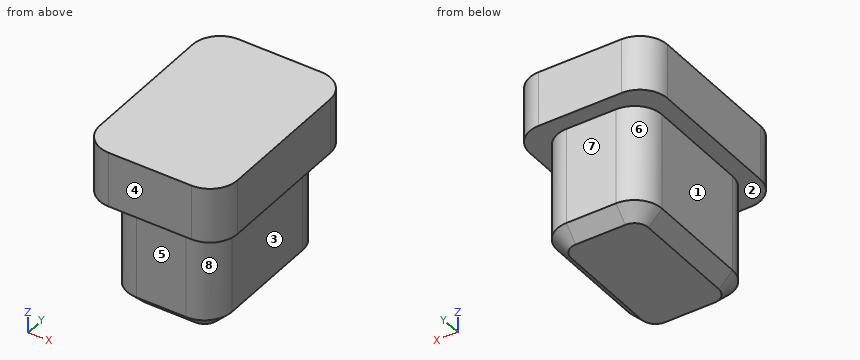
Autodesk Inventor part; units mm, degrees
ref_plane "YZ Plane" through (0, 0, 0) normal (1, 0, 0) x (0, 1, 0)
ref_plane "XZ Plane" through (0, 0, 0) normal (0, 1, 0) x (-1, 0, 0)
ref_plane "XY Plane" through (0, 0, 0) normal (0, 0, 1) x (1, 0, 0)
sketch "Sketch1" plane through (0, 0, 0) normal (0, 0, 1) x (1, 0, 0)
  line L0 (-0.9, 2.9) -> (0.9, 2.9)
  line L1 (1.9, 1.9) -> (1.9, -1.9)
  line L2 (0.9, -2.9) -> (-0.9, -2.9)
  line L3 (-1.9, -1.9) -> (-1.9, 1.9)
  arc A0 (1.9, 1.9) -> (0.9, 2.9) centre (0.9, 1.9) ccw
  arc A1 (0.9, -2.9) -> (1.9, -1.9) centre (0.9, -1.9) ccw
  arc A2 (-1.9, -1.9) -> (-0.9, -2.9) centre (-0.9, -1.9) ccw
  arc A3 (-0.9, 2.9) -> (-1.9, 1.9) centre (-0.9, 1.9) ccw
  point P0 (0, 0)
  point P1 (0, 2.9)
  point P2 (-1.9, 0)
  dimension "d1" = 3.8
  dimension "d2" = 5.8
  dimension "d3" = 1
extrude "Extrusion1" add sketch "Sketch1" along normal blind 4
sketch "Sketch2" plane through (0, 0, 4) normal (0, 0, 1) x (1, 0, 0)
  line L0 (-1.5, 3.5) -> (1.5, 3.5)
  line L1 (2.5, 2.5) -> (2.5, -2.5)
  line L2 (1.5, -3.5) -> (-1.5, -3.5)
  line L3 (-2.5, -2.5) -> (-2.5, 2.5)
  arc A0 (2.5, 2.5) -> (1.5, 3.5) centre (1.5, 2.5) ccw
  arc A1 (-2.5, -2.5) -> (-1.5, -3.5) centre (-1.5, -2.5) ccw
  arc A2 (1.5, -3.5) -> (2.5, -2.5) centre (1.5, -2.5) ccw
  arc A3 (-1.5, 3.5) -> (-2.5, 2.5) centre (-1.5, 2.5) ccw
  point P0 (0, 0)
  point P1 (-2.5, 3.5)
  point P2 (2.5, -3.5)
  point P3 (2.5, 3.5)
  point P4 (0, 3.5)
  point P5 (2.5, 0)
  dimension "d6" = 5
  dimension "d7" = 7
  dimension "d9" = 1
extrude "Extrusion2" add sketch "Sketch2" along normal blind 2
chamfer "Chamfer1" distance 0.5 angle 45 8 edges at (-1.9, 0, 0) (-1.6071, -2.6071, 0) (0, -2.9, 0) (1.6071, -2.6071, 0) (1.9, 0, 0) (1.6071, 2.6071, 0) (0, 2.9, 0) (-1.6071, 2.6071, 0)
properties part number "Button_Extender"
The model under review builds one solid part; all positions refer to its coordinate system, in mm. Face numbers are marked on the shaded views. A direction names the side the tool comes from. Round coordinates to 2 decimals unless told otherwise and drop trailing zeros. Order: outer loops, then holes, each group sorted by start corner. A loop starts at its lowest first (then second) coordinate and runs counter-clockwise, first axis right, second up.
(1) Take a section at A-A, the plane z = 4.4. State the section outline as (x, y) points, plus the area to 3 significant figures.
Working result:
outline: (-2.5, -2.5) arc R1 ccw to (-1.5, -3.5) - (1.5, -3.5) arc R1 ccw to (2.5, -2.5) - (2.5, 2.5) arc R1 ccw to (1.5, 3.5) - (-1.5, 3.5) arc R1 ccw to (-2.5, 2.5) - close
area: 34.1 mm2
(2) Take a section at C-C, the plane x = 0.8. State the section outline as (y, z) points, plus the area to 4 significant figures.
Working result:
outline: (-3.5, 4) - (-2.9, 4) - (-2.9, 0.5) - (-2.4, 0) - (2.4, 0) - (2.9, 0.5) - (2.9, 4) - (3.5, 4) - (3.5, 6) - (-3.5, 6) - close
area: 36.95 mm2
(3) For P1, Ø3, axis at y = -1, z = 1, coming from the -X side; P2, Ø0.5, axis at x = -0.5, z = 2.5, coming from the +Y side; P3, Ø1.4, axis at x = -0.5, z = 2.5, coming from the -Y side; P4, Ø2, axis at x = -2, y = 0, coming from the -Z side, all flat-tipped, find the tip position at first contact; note any pin that passes through.
Working result:
P1: stops at x = -1.9
P2: stops at y = 2.9
P3: stops at y = -2.9
P4: stops at z = 0
(4) Take a section at B-B, the plane y = -1.5. State the section outline as (x, z) points.
Working result:
outline: (-2.5, 4) - (-1.9, 4) - (-1.9, 0.5) - (-1.4, 0) - (1.4, 0) - (1.9, 0.5) - (1.9, 4) - (2.5, 4) - (2.5, 6) - (-2.5, 6) - close
(5) Mouldability with a two-part tool opening along X and no side actions: class the marked faces 6, 7 and 8 as released by +X, released by -X, zero draft, split by the parting line, or undercut.
Working result:
face 6: released by -X
face 7: zero draft
face 8: released by +X
(6) Wall thickness on L1, parallel to X at y = -0.25, z = 1.6; L2, parallel to Z at x = -2, y = -1.75; L3, parallel to Y at x = -0.65, z = 0.9: over which ranges is each line inside the solid? List them lowest first.
Working result:
L1: x = -1.9 to 1.9
L2: z = 4 to 6
L3: y = -2.9 to 2.9
(7) Take a section at D-D, the plane z = 3.7. State the section outline as (x, y) points, plus the area to 3 significant figures.
Working result:
outline: (-1.9, -1.9) arc R1 ccw to (-0.9, -2.9) - (0.9, -2.9) arc R1 ccw to (1.9, -1.9) - (1.9, 1.9) arc R1 ccw to (0.9, 2.9) - (-0.9, 2.9) arc R1 ccw to (-1.9, 1.9) - close
area: 21.2 mm2
(8) Tool access review of the marked faces 1, 2, 3, 4 and 5: name each direction out of +Z, -Z, +X, -X, +Y, -Y from which nothing blocks a thin tool from reaching the whole face with its end or side.
Working result:
face 1: -Z, -X, +Y, -Y
face 2: -Z
face 3: -Z, +X, +Y, -Y
face 4: +Z, -Z, +X, -X, -Y
face 5: -Z, +X, -X, -Y
